The model under review builds one solid part; all positions refer to its coordinate system, in mm. Face numbers are marked on the shaded views. A direction names the side the tool comes from. Round coordinates to 2 decimals unless told otherwise and drop trailing zeros. Write each loop counter-clockwise with the first axis right and the second up, starting at its lowest first coordinate (ties: lowest second). Pieces come first, ordered by that corner, then holes. Notation, with made-up numbers: M 17,36.5 L 62,36.5 A21 ccw 62,51.5 Z; hole C -21.75,-19 d10. An arc over 180 degrees is marked long. One line per item, written item: value. Start each with the question number.
1) Take a section at B-B, the plane y = -3.75. Write out the cut boundary in (x, z).
2) Take a section at D-D, the plane y = -8.25. Write out the cut boundary in (x, z).
3) Mouldability with a two-part tool opening along Y and no side actions: class the marked faces 1, 2, 3 and 4 as +Y half, -Y half, draft (parallel to the pull), parting line (faces both ways), or undercut.
4) Take a section at C-C, the plane x = -6. Write out the cut boundary in (y, z), and give its area (3 significant figures).
5) For P1, Ø1, axis at y = -3, z = 7, coming from the +X side; P2, Ø0.6, axis at x = -0.5, z = 11.5, coming from the +Y side; P3, Ø4, axis at x = -3.5, y = -8.5, coming from the -Z side, all flat-tipped, find the tip position at first contact; note any pin that passes through.
6) Take a section at A-A, the plane z = 4.25. Write out the cut boundary in (x, y).
7) Tool access review of the marked faces 5, 6, 7, 8 and 9: name each direction out of +Z, -Z, +X, -X, +Y, -Y from which nothing blocks a thin tool from reaching the whole face with its end or side.
8) Wall thickness on probe 1 along X at (y, z) = (7.75, 4.5); probe 2 along Y at (x, z) = (-7.5, 2.5); probe 3 along Z at (x, y) = (-1.75, -1.75): over which ranges is each line inside the solid? List them lowest first.
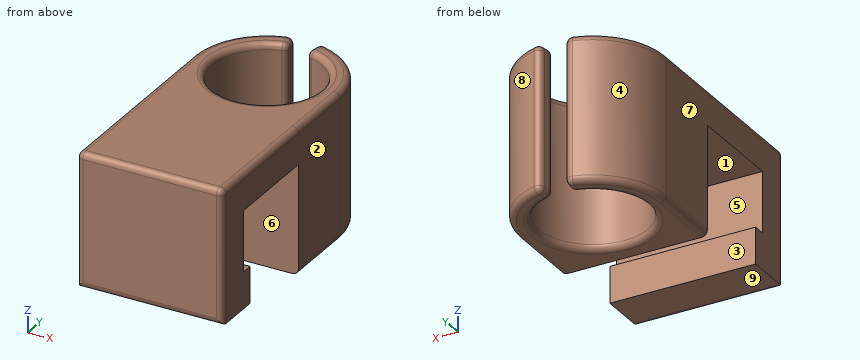
from build123d import *

# Parameters (mm, degrees)
F1_DEPTH = 12
F2_R     = 0.5
F4_DEPTH = 12
F5_R     = 0.5


with BuildPart() as f1:
    # F0 (on Top) → F1 (new body)
    with BuildSketch(Plane.XY):
        with BuildLine():
            Line((-12, 0), (0, 0))
            Line((0, 0), (0, 6))
            ThreePointArc((0, 6), (-1.403733, 9.856726), (-4.958111, 11.908847))
            Line((-4.958111, 11.908847), (-5.218583, 10.431635))
            ThreePointArc((-5.218583, 10.431635), (-6, 1.5), (-6.781417, 10.431635))
            Line((-6.781417, 10.431635), (-7.041889, 11.908847))
            ThreePointArc((-7.041889, 11.908847), (-10.596267, 9.856726), (-12, 6))
            Line((-12, 6), (-12, 0))
        make_face()
    extrude(amount=F1_DEPTH)

    # F2
    f2_edges = [f1.edges().sort_by_distance(p)[0] for p in [
        (-6.781417, 10.431635, 6),
        (-7.041889, 11.908847, 6),
        (-5.218583, 10.431635, 6),
        (-4.958111, 11.908847, 6),
        (-10.596267, 9.856726, 0),
        (-10.596267, 9.856726, 12),
        (-12, 3, 0),
        (-12, 3, 12),
        (-1.403733, 9.856726, 0),
        (0, 3, 0),
        (-1.403733, 9.856726, 12),
        (0, 3, 12),
        (-6.911653, 11.170241, 0),
        (-5.088347, 11.170241, 0),
        (-6.911653, 11.170241, 12),
        (-5.088347, 11.170241, 12),
        (-6, 1.5, 12),
        (-6, 1.5, 0),
    ]]
    fillet(f2_edges, radius=F2_R)

    # F3 (on face) → F4 (join)
    with BuildSketch(Plane.YZ):
        Polygon((0, 11.5), (0, 12), (-11, 12), (-11, 1), (-7, 1), (-7, 4), (-8, 4), (-8, 9), (0, 9), align=None)
    extrude(amount=-F4_DEPTH)

    # F5
    f5_edges = [f1.edges().sort_by_distance(p)[0] for p in [
        (0, -5.5, 12),
        (-12, -5.5, 12),
        (-12, -11, 6.5),
        (-6, -11, 12),
        (0, -11, 6.5),
        (-6, -11, 1),
    ]]
    fillet(f5_edges, radius=F5_R)


solid = f1.part
Checked values:
1. outline: M -12,9 L 0,9 L 0,11.5 A0.5 ccw -0.5,12 L -11.5,12 A0.5 ccw -12,11.5 Z
2. outline: M -12,1 L 0,1 L 0,11.5 A0.5 ccw -0.5,12 L -11.5,12 A0.5 ccw -12,11.5 Z
3. face 1: undercut
3. face 2: draft
3. face 3: undercut
3. face 4: +Y half
4. outline: M -11,1.5 A0.5 ccw -10.5,1 L -7,1 L -7,4 L -8,4 L -8,9 L 0,9 L 0,0 L 1,0 A0.5 ccw 1.5,0.5 L 1.5,11.5 A0.5 ccw 1,12 L -10.5,12 A0.5 ccw -11,11.5 Z
4. area: 77.8 mm2
5. P1: passes through
5. P2: stops at y = 8.99
5. P3: stops at z = 1
6. outline: M -12,-10.5 A0.5 ccw -11.5,-11 L -0.5,-11 A0.5 ccw 0,-10.5 L 0,-8 L -12,-8 Z; M -12,0 L 0,0 L 0,6 A6 ccw -4.43,11.79 A0.5 ccw -5.05,11.39 L -5.14,10.9 A0.5 ccw -4.78,10.33 A4.5 cw long -7.22,10.33 A0.5 ccw -6.86,10.9 L -6.95,11.39 A0.5 ccw -7.57,11.79 A6 ccw -12,6 Z
7. face 5: +X, -X
7. face 6: -Z, +X, -X
7. face 7: +Z, -Z, -X, +Y, -Y
7. face 8: +Z, -Z, +X, +Y
7. face 9: -Z, +X, -X, -Y
8. probe 1: x = -11.74 to -10.15, -1.85 to -0.26
8. probe 2: y = -11 to -7, 0 to 1.76, 10.24 to 11.8
8. probe 3: z = 9 to 12
